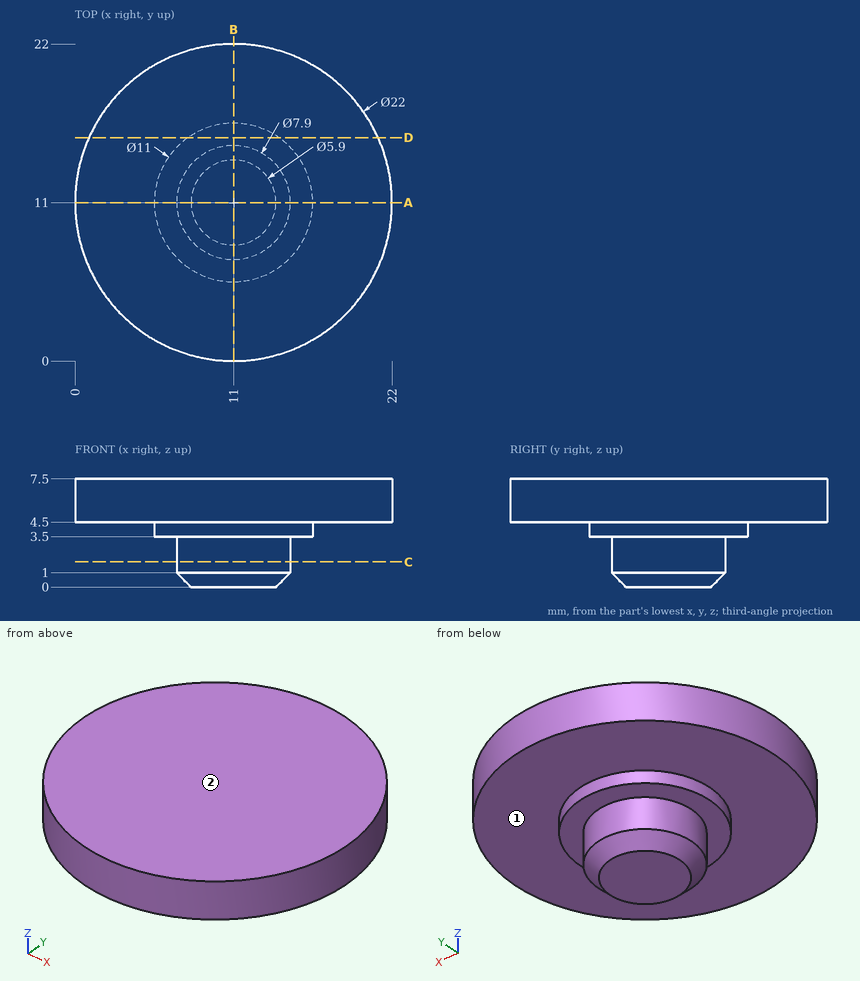
Geometry: see drawing. Coordinates: mm, zero at the bounding-box minimum. A direction names the side the tool comes from. Coordinates: 2 decimals unless noted, no trailing zeros. Order: outer loops, then holes, each group sorted by start corner. A loop starts at its lowest first (then second) coordinate and runs counter-clockwise, first axis right, second up. Notation, with made-up numbers: M -16,-15.5 L 43,-15.5 A22 cw 43,16.5 Z; hole C -6,71.5 d9. An arc over 180 degrees is marked long. Answer as CSV lines item,"result".
1. Section D-D (y = 15.5). Return the cut outline in (x, z), then the cut area to 3 significant figures.
Reported:
outline,"M 0.96,4.5 L 7.84,4.5 L 7.84,3.5 L 14.16,3.5 L 14.16,4.5 L 21.04,4.5 L 21.04,7.5 L 0.96,7.5 Z"
area,"66.5 mm2"
2. Section A-A (y = 11). Return the cut outline in (x, z).
Reported:
outline,"M 0,4.5 L 5.5,4.5 L 5.5,3.5 L 7.05,3.5 L 7.05,1 L 8.05,0 L 13.95,0 L 14.95,1 L 14.95,3.5 L 16.5,3.5 L 16.5,4.5 L 22,4.5 L 22,7.5 L 0,7.5 Z"
3. Section C-C (z = 1.75). Return the cut outline in (x, y).
Reported:
outline,"C 11,11 d7.9"
4. First-contact query: P1, Ø1.5, axis at x = 5, y = 8, coming from the -Z side; P2, Ø4, axis at x = 17, z = 5, coming from the +Y side. Flat tips, straight axial feed; report the tip coordinate or a pass-through.
Reported:
P1,"z = 4.5"
P2,"y = 21.25"
5. Material intervals for line 1 (Z direction, x = 6, y = 7.5); line 2 (Z direction, x = 10, y = 6.5); line 3 (Y direction, x = 12.75, z = 7.25), sorted ascending. Write a range as from..to.
Reported:
line 1,"4.5..7.5"
line 2,"3.5..7.5"
line 3,"0.14..21.86"
6. Access query for the marked faces 1 and 2. Directions: +Z, -Z, +X, -X, +Y, -Y. A direction counts if a zero-diameter tool reaches every point of the face in a straight line with its end or side. Return the directions, or none.
Reported:
face 1,"-Z"
face 2,"+Z, +X, -X, +Y, -Y"
